```python
from build123d import *

# Parameters (mm, degrees)
SKETCH1_W           = 50
SKETCH1_H           = 10
BOSS_EXTRUDE1_DEPTH = 2
CUT_EXTRUDE1_DEPTH  = 3


with BuildPart() as part:
    # Sketch1 → Boss-Extrude1 (new body)
    with BuildSketch(Plane(origin=(0, 0, 0), x_dir=(1, 0, 0), z_dir=(0, 1, 0))):
        with Locations((25, 5)):
            Rectangle(SKETCH1_W, SKETCH1_H)
        with BuildLine():
            Line((3.15, 7.034698995), (3.15, 2.965301005))
            ThreePointArc((3.15, 2.965301005), (5, 2.25), (6.85, 2.965301005))
            Line((6.85, 2.965301005), (6.85, 7.034698995))
            ThreePointArc((6.85, 7.034698995), (5, 7.75), (3.15, 7.034698995))
        make_face(mode=Mode.SUBTRACT)
        with BuildLine():
            Line((11.125, 7.045727255), (11.125, 2.954272745))
            ThreePointArc((11.125, 2.954272745), (13, 2.225), (14.875, 2.954272745))
            Line((14.875, 2.954272745), (14.875, 7.045727255))
            ThreePointArc((14.875, 7.045727255), (13, 7.775), (11.125, 7.045727255))
        make_face(mode=Mode.SUBTRACT)
        with BuildLine():
            Line((19.1, 7.05669638), (19.1, 2.94330362))
            ThreePointArc((19.1, 2.94330362), (21, 2.2), (22.9, 2.94330362))
            Line((22.9, 2.94330362), (22.9, 7.05669638))
            ThreePointArc((22.9, 7.05669638), (21, 7.8), (19.1, 7.05669638))
        make_face(mode=Mode.SUBTRACT)
        with BuildLine():
            Line((27.075, 7.067607313), (27.075, 2.932392687))
            ThreePointArc((27.075, 2.932392687), (29, 2.175), (30.925, 2.932392687))
            Line((30.925, 2.932392687), (30.925, 7.067607313))
            ThreePointArc((30.925, 7.067607313), (29, 7.825), (27.075, 7.067607313))
        make_face(mode=Mode.SUBTRACT)
        with BuildLine():
            Line((38.95, 2.921539031), (38.95, 7.078460969))
            ThreePointArc((38.95, 7.078460969), (37, 7.85), (35.05, 7.078460969))
            Line((35.05, 7.078460969), (35.05, 2.921539031))
            ThreePointArc((35.05, 2.921539031), (37, 2.15), (38.95, 2.921539031))
        make_face(mode=Mode.SUBTRACT)
        with BuildLine():
            Line((46.975, 2.910741758), (46.975, 7.089258242))
            ThreePointArc((46.975, 7.089258242), (45, 7.875), (43.025, 7.089258242))
            Line((43.025, 7.089258242), (43.025, 2.910741758))
            ThreePointArc((43.025, 2.910741758), (45, 2.125), (46.975, 2.910741758))
        make_face(mode=Mode.SUBTRACT)
    extrude(amount=BOSS_EXTRUDE1_DEPTH)

    # Sketch2 → Cut-Extrude1 (cut, through all)
    with BuildSketch(Plane(origin=(0, 2, 0), x_dir=(1, 0, 0), z_dir=(0, 1, 0))):
        Polygon((0, 7), (3, 10), (0, 10), align=None)
    extrude(amount=-CUT_EXTRUDE1_DEPTH, mode=Mode.SUBTRACT)


solid = part.part
```
Here's how the part is built. I have some questions about the finished solid (model axes, mm). A direction names the side the tool comes from. Round coordinates to 2 decimals unless told otherwise and drop trailing zeros. Loops run counter-clockwise (first coordinate to the right, second up) from the corner with the lowest first, then second, coordinate; pieces in that order, holes last.
1. Suppose I cut it at D-D, the plane z = -9. Please give me the cut outline in (x, y).
Answers:
outline: (2, 0) - (50, 0) - (50, 2) - (2, 2) - close
2. Suppose I cut it at A-A, the plane z = -6.25. Please give me the cut outline in (x, y) (3 decimals).
Answers:
outline: (0, 0) - (3.15, 0) - (3.15, 2) - (0, 2) - close; (6.85, 0) - (11.125, 0) - (11.125, 2) - (6.85, 2) - close; (14.875, 0) - (19.1, 0) - (19.1, 2) - (14.875, 2) - close; (22.9, 0) - (27.075, 0) - (27.075, 2) - (22.9, 2) - close; (30.925, 0) - (35.05, 0) - (35.05, 2) - (30.925, 2) - close; (38.95, 0) - (43.025, 0) - (43.025, 2) - (38.95, 2) - close; (46.975, 0) - (50, 0) - (50, 2) - (46.975, 2) - close
3. If I drill on probe 1 along Z at (x, y) = (29.5, 1.9); probe 2 along Z at (x, y) = (28, 0.9); probe 3 along X at (y, z) = (0.8, -9.25), over which ranges is the centre line in solid material (lowest first)?
Answers:
probe 1: z = -10 to -7.78, -2.22 to 0
probe 2: z = -10 to -7.64, -2.36 to 0
probe 3: x = 2.25 to 50
4. For faces 1 (the face through (26, 1, -10)), 2 (the face through (43.025, 1, -5)), which set-ups out of +Z, -Z, +X, -X, +Y, -Y let a thin tool reach every point of the face, with its end or its side?
Answers:
face 1: -Z, +X, -X, +Y, -Y
face 2: +Y, -Y
5. Suppose I cut it at C-C, the plane y = 0.55. Give the number of separate pieces and of enclosed holes in the cut face, and give its area (3 significant figures).
Answers:
separate pieces: 1
enclosed holes: 6
area: 377 mm2
6. Suppose I cut it at B-B, the plane x = 37. Please give me the cut outline in (y, z), and give its area (3 significant figures).
Answers:
outline: (0, -10) - (2, -10) - (2, -7.85) - (0, -7.85) - close; (0, -2.15) - (2, -2.15) - (2, 0) - (0, 0) - close
area: 8.60 mm2
